```python
from build123d import *

# Parameters (mm, degrees)
F0_W          = 7
F0_H          = 9
F0_R          = 1.85
F1_DEPTH      = 5
F5_ANGLE_BACK = 20
F5_ANGLE      = 40
F6_W          = 1.6
F6_H          = 1.8669135356
F6_H_2        = 10
F7_DEPTH      = 5
F8_W          = 7
F8_H          = 1.5
F9_DEPTH      = 4
F10_W         = 0.2
F10_H         = 4
F11_DEPTH     = 25


with BuildPart() as f1:
    # F0 (on Top) → F1 (new body)
    with BuildSketch(Plane.XY):
        with Locations((3.5, -4.5)):
            Rectangle(F0_W, F0_H)
        with Locations((4, -4.5)):
            Circle(F0_R, mode=Mode.SUBTRACT)
    extrude(amount=F1_DEPTH)

    # F3 (on offset) → F5 (revolve)
    with BuildSketch(Plane.XZ.offset(4.5), mode=Mode.PRIVATE) as f5_sk:
        with BuildLine():
            Line((0.5, 5), (0, 5))
            Line((0, 5), (-0.5, 5))
            Line((-0.5, 5), (-0.5, 0))
            add(Edge.make_bspline(
                [(-0.5, 0), (-0.7940392474, -1.8718490053), (-2.3993364256, -10.2948176613), (-9.1089938236, -15.538515672), (-10.3149545762, -17)],
                knots=[0, 0, 0, 0, 0.5, 1, 1, 1, 1], degree=3))
            ThreePointArc((-10.3149545762, -17), (-10.1685444147, -17.5464101615), (-9.6221342532, -17.4))
            add(Edge.make_bspline(
                [(-9.6221342532, -17.4), (-8.3348966668, -15.9883498775), (-1.3566520207, -10.8349816991), (0.0036717937, -2.0199950425), (0.5, 0)],
                knots=[0, 0, 0, 0, 0.4942337757, 1, 1, 1, 1], degree=3))
            Line((0.5, 0), (0.5, 5))
        make_face()
    revolve(f5_sk.sketch.rotate(Axis((-20, -4.5, 1.4354154991), (0, 0, -1)), -F5_ANGLE_BACK), axis=Axis((-20, -4.5, 1.4354154991), (0, 0, -1)), revolution_arc=F5_ANGLE)

    # F6 (on face) → F7 (cut)
    with BuildSketch(Plane.XY.offset(5)):
        with Locations((0.8, -9.9334567678)):
            Rectangle(F6_W, F6_H)
        with Locations((0.8, 5)):
            Rectangle(F6_W, F6_H_2)
    extrude(amount=-F7_DEPTH, mode=Mode.SUBTRACT)

    # F8 (on face) → F9 (join)
    with BuildSketch(Plane.XY.offset(5)):
        with Locations((3.5, -0.75)):
            Rectangle(F8_W, F8_H)
        with Locations((3.5, -8.25)):
            Rectangle(F8_W, F8_H)
    extrude(amount=F9_DEPTH)

    # F10 (on face) → F11 (cut)
    with BuildSketch(Plane.YZ.offset(7)):
        with Locations((-7.6, 7)):
            Rectangle(F10_W, F10_H)
        with Locations((-8.9, 7)):
            Rectangle(F10_W, F10_H)
        with Locations((-0.1, 7)):
            Rectangle(F10_W, F10_H)
        with Locations((-1.4, 7)):
            Rectangle(F10_W, F10_H)
    extrude(amount=-F11_DEPTH, mode=Mode.SUBTRACT)


solid = f1.part
```
CAD build for the part. Positions are in the model's coordinates, mm. A direction names the side the tool comes from. Give positions to 0.01 mm unless a question says otherwise; leave off trailing zeros. Order: outer loops, then holes, each group sorted by start corner. A loop starts at its lowest first (then second) coordinate and runs counter-clockwise, first axis right, second up.
(1) Flat gauge pins, fed straight in: pin 1 (3 mm diameter, centred on x = 4.5, z = 6, fed in from -Y); pin 2 (4 mm diameter, centred on x = 4.5, z = 2.5, fed in from +Y); pin 3 (8 mm diameter, centred on y = -7.5, z = -9, fed in from +X). Where does each tip first touch, or does it go through?
(2) Tool access for faces 1 (the flat face through (4, -8.8, 7)), 2 (the flat face through (3, -9, 2)), 3 (the flat face through (4, -7.7, 7)): list every direction of +Z, -Z, +X, -X, +Y, -Y with a clear straight run to the whole face (end or side of a thin tool).
(3) Drill centre lines: L1, parallel to Y at x = 4, z = 2.55; L2, parallel to Z at x = 2, y = -6; L3, parallel to X at y = -1.25, z = 7. Where is each one in solid material? Low to high.
(4) Mould opens along X. For faces 4 (the flat face through (0, -1, 7)), 5 (the cylindrical face through (-0.323, -10.25, 2.535)), 6 (the cylindrical face through (3.759, -2.666, 2.465)), 7 (the flat face through (3, 0, 2)) say: released by +X, released by -X, zero draft, split by the parting line, or undercut.
(5) Saw through at A-A, the plane z = 3.5. Give the cut face in (x, y).
(6) Saw through at B-B, the plane x = 4. Give the cut face in (y, z).
Results found:
1. pin 1: stops at y = -9
1. pin 2: stops at y = 0
1. pin 3: stops at x = -0.84
2. face 1: +Z, +X, -X, -Y
2. face 2: +Z, -Z, +X, -Y
2. face 3: +Z, +X, -X
3. L1: y = -9 to -6.35, -2.65 to 0
3. L2: z = 0 to 5
3. L3: x = 0 to 7
4. face 4: released by -X
4. face 5: released by +X
4. face 6: undercut
4. face 7: zero draft
5. outline: (-1.68, -11.17) - (-0.74, -11.51) arc R20.5 ccw to (0, -9) - (7, -9) - (7, 0) - (0, 0) arc R20.5 ccw to (-0.74, 2.51) - (-1.68, 2.17) arc R19.5 cw to start; hole circle Ø3.7 at (4, -4.5)
6. outline: (-9, 0) - (-6.35, 0) - (-6.35, 5) - (-7.7, 5) - (-7.7, 9) - (-8.8, 9) - (-8.8, 5) - (-9, 5) - close; (-2.65, 0) - (0, 0) - (0, 5) - (-0.2, 5) - (-0.2, 9) - (-1.3, 9) - (-1.3, 5) - (-2.65, 5) - close
